```python
from build123d import *

# Parameters (mm, degrees)
SKETCH1_R          = 4.7625
SKETCH1_R_2        = 3.175
EXTRUDE1_DEPTH     = 15.875
SKETCH2_R          = 3.175
EXTRUDE2_DEPTH     = 3.175
SKETCH3_R          = 4.7625
SKETCH3_R_2        = 3.175
EXTRUDE3_DEPTH     = 5.08
SKETCH4_R          = 6.35
SKETCH4_R_2        = 4.7625
CUT_EXTRUDE1_DEPTH = 1.5875
SKETCH5_R          = 5.588
SKETCH5_R_2        = 4.7625
EXTRUDE4_DEPTH     = 6.35


with BuildPart() as part:
    # Sketch1 → Extrude1 (new body)
    with BuildSketch(Plane(origin=(0, 0, 0), x_dir=(1, 0, 0), z_dir=(0, 1, 0))):
        Circle(SKETCH1_R)
        Circle(SKETCH1_R_2, mode=Mode.SUBTRACT)
    extrude(amount=EXTRUDE1_DEPTH)

    # Sketch2 → Extrude2 (add)
    with BuildSketch(Plane.XZ):
        Polygon((7.973928905, 4.60375), (7.973928905, -4.60375), (0, -9.2075), (-7.973928905, -4.60375), (-7.973928905, 4.60375), (0, 9.2075), align=None)
        Circle(SKETCH2_R, mode=Mode.SUBTRACT)
    extrude(amount=EXTRUDE2_DEPTH)

    # Sketch3 → Extrude3 (add)
    with BuildSketch(Plane.XZ.offset(3.175)):
        Circle(SKETCH3_R)
        Circle(SKETCH3_R_2, mode=Mode.SUBTRACT)
    extrude(amount=EXTRUDE3_DEPTH)

    # Sketch4 → Cut-Extrude1 (cut)
    with BuildSketch(Plane.XZ.offset(3.175)):
        Circle(SKETCH4_R)
        Circle(SKETCH4_R_2, mode=Mode.SUBTRACT)
    extrude(amount=-CUT_EXTRUDE1_DEPTH, mode=Mode.SUBTRACT)

    # Sketch5 → Extrude4 (add)
    with BuildSketch(Plane(origin=(0, 15.875, 0), x_dir=(-1, 0, 0), z_dir=(0, 1, 0))):
        Circle(SKETCH5_R)
        Circle(SKETCH5_R_2, mode=Mode.SUBTRACT)
    extrude(amount=-EXTRUDE4_DEPTH)

    # Sketch7 → Cut-Revolve1 (revolve, cut)
    with BuildSketch(Plane(origin=(0, 0, 0), x_dir=(0, 0, -1), z_dir=(1, 0, 0))):
        Polygon((-5.588, 9.525), (-4.7625, 15.875), (-5.588, 15.875), align=None)
    revolve(axis=Axis((0, 15.875, 0), (0, -1, 0)), mode=Mode.SUBTRACT)


solid = part.part
```
Input: part model. Units: mm. Frame: model coordinates. A direction names the side the tool comes from. Coordinates: 2 decimals unless noted, no trailing zeros. Answer in a Markdown table with one row per item.
(1) Mould query, pull axis Y, two halves, no side actions, for faces 4 (the face through (-3.78, 4.7, 2.9)), 5 (the face through (1, -1.588, 5)), 6 (the face through (-3.93, -1.57, -6.94)), 7 (the face through (-3, 0, -4)). Classes: pulls with the +Y half, pulls with the -Y half, needs draft (parallel to the pull), parting line crosses it, or undercut.
Model answer:
| item | result |
|---|---|
| face 4 | undercut |
| face 5 | pulls with the -Y half |
| face 6 | needs draft |
| face 7 | undercut |
(2) Cut plane A-A on y = -2.5. Count the separate pieces of the cut face and the enclosed holes in it, plus the area to 3 significant figures.
Model answer:
| item | result |
|---|---|
| separate pieces | 2 |
| enclosed holes | 2 |
| area | 133 mm² |
(3) Set-up query: faces 1 (the face through (-4, 9.525, 3)), 2 (the face through (-3.78, -4.97, -2.9)), 3 (the face through (4, -1.6, -6.9)). Return all of +Z, -Z, +X, -X, +Y, -Y with unobstructed straight access to the full face (end or side cutting, diameter ignored); none if empty.
Model answer:
| item | result |
|---|---|
| face 1 | none |
| face 2 | -Y |
| face 3 | -Z, +X, +Y, -Y |
(4) Material intervals for L1, parallel to X at y = 8.75, z = 0 (1 decimal); L2, parallel to Y at x = 0.5, z = 7.25 (3 decimals), sorted ascending. Write a range as from..to.
Model answer:
| item | result |
|---|---|
| L1 | x = -4.8..-3.2, 3.2..4.8 |
| L2 | y = -3.175..0 |
(5) Pin query (flat end, axial travel): P1, Ø5, axis at x = -0.5, y = 12, coming from the -Z side; P2, Ø3, axis at y = 2, z = 0.5, coming from the -X side; P3, Ø8, axis at y = 12, z = -5.5, coming from the -X side. Return the tip coordinate at first contact, or that it passes through.
Model answer:
| item | result |
|---|---|
| P1 | stops at z = -5.59 |
| P2 | stops at x = -4.76 |
| P3 | stops at x = -5.16 |
